Build history of the part. All positions in model axes, mm. A direction names the side the tool comes from. Coordinates: 2 decimals unless noted, no trailing zeros. Order: outer loops, then holes, each group sorted by start corner. A loop starts at its lowest first (then second) coordinate and runs counter-clockwise, first axis right, second up. Notation, with made-up numbers: M -8,-25.5 L -4,-25.5 A21 cw -4,-4.5 Z; hole C 81,9.25 d11. An arc over 180 degrees is marked long. Use a Markdown table: item, result. Add a question column.
from build123d import *

# Parameters (mm, degrees)
F0_R     = 57.15
F1_DEPTH = 14.224
F3_DEPTH = 30.226
F4_R     = 7.112
F5_DEPTH = 0.127


with BuildPart() as f1:
    # F0 (on Top) → F1 (new body)
    with BuildSketch(Plane.XY):
        Circle(F0_R)
        with BuildLine():
            ThreePointArc((0, -29.464), (5.0289434278, -31.5470565722), (7.112, -36.576))
            ThreePointArc((7.112, -36.576), (-5.0289434278, -41.6049434278), (0, -29.464))
        make_face(mode=Mode.SUBTRACT)
        with BuildLine():
            ThreePointArc((-24.5637451688, 18.288), (-24.8060806923, 16.4472789512), (-25.5165724971, 14.732))
            ThreePointArc((-25.5165724971, 14.732), (-38.5454096454, 20.1287210488), (-24.5637451688, 18.288))
        make_face(mode=Mode.SUBTRACT)
        with BuildLine():
            ThreePointArc((15.875, 0), (11.2253201513, -11.2253201513), (0, -15.875))
            ThreePointArc((0, -15.875), (-13.7481532851, -7.9375), (-13.7481532851, 7.9375))
            ThreePointArc((-13.7481532851, 7.9375), (0, 15.875), (13.7481532851, 7.9375))
            ThreePointArc((13.7481532851, 7.9375), (15.3340724923, 4.108752341), (15.875, 0))
        make_face(mode=Mode.SUBTRACT)
        with BuildLine():
            ThreePointArc((38.7877451688, 18.288), (33.5164662176, 11.4183355234), (25.5165724971, 14.732))
            ThreePointArc((25.5165724971, 14.732), (29.8350241201, 25.1576644766), (38.7877451688, 18.288))
        make_face(mode=Mode.SUBTRACT)
    extrude(amount=F1_DEPTH)

    # F2 (on face) → F3 (join)
    with BuildSketch(Plane.XY.offset(14.224)):
        with BuildLine():
            ThreePointArc((-17.1202854359, -34.0368304428), (-32.4337237695, -19.9915872918), (-38.1, 0))
            Line((-38.1, 0), (-50.8, 0))
            ThreePointArc((-50.8, 0), (-43.244965026, -26.6554497224), (-22.8270472479, -45.3824405904))
            Line((-22.8270472479, -45.3824405904), (-17.1202854359, -34.0368304428))
        make_face()
        with BuildLine():
            ThreePointArc((-20.7239090963, 31.9707615137), (0, 38.1), (20.7239090963, 31.9707615137))
            Line((20.7239090963, 31.9707615137), (27.6318787951, 42.6276820183))
            ThreePointArc((27.6318787951, 42.6276820183), (0, 50.8), (-27.6318787951, 42.6276820183))
            Line((-27.6318787951, 42.6276820183), (-20.7239090963, 31.9707615137))
        make_face()
        with BuildLine():
            ThreePointArc((38.1, 0), (32.6002459501, -19.7188732942), (17.6887682944, -33.7448881496))
            Line((17.6887682944, -33.7448881496), (23.5850243925, -44.9931841994))
            ThreePointArc((23.5850243925, -44.9931841994), (43.4669946002, -26.2918310589), (50.8, 0))
            Line((50.8, 0), (38.1, 0))
        make_face()
    extrude(amount=F3_DEPTH)

    # F4 (on face) → F5 (cut)
    with BuildSketch(Plane.XY.offset(14.224)):
        with BuildLine():
            ThreePointArc((-20.7239090963, 31.9707615137), (-47.4729372454, 10.6979144605), (-14.1497451688, 18.288))
            ThreePointArc((-14.1497451688, 18.288), (-15.8785530923, 25.8780855395), (-20.7239090963, 31.9707615137))
        make_face()
        with Locations((-31.6757451688, 18.288)):
            Circle(F4_R, mode=Mode.SUBTRACT)
        with BuildLine():
            ThreePointArc((49.2017451688, 18.288), (39.2658307083, 34.0851920765), (20.7239090963, 31.9707615137))
            ThreePointArc((20.7239090963, 31.9707615137), (24.0856596293, 2.4908079235), (49.2017451688, 18.288))
        make_face()
        with Locations((31.6757451688, 18.288)):
            Circle(F4_R, mode=Mode.SUBTRACT)
        with BuildLine():
            ThreePointArc((-17.4173370009, -34.6273985025), (-0.9758144603, -54.0748131637), (17.526, -36.576))
            ThreePointArc((17.526, -36.576), (1.3253891442, -19.1001875835), (-17.325537101, -33.9328125))
            ThreePointArc((-17.325537101, -33.9328125), (-17.2229897955, -33.9849764235), (-17.1202854359, -34.0368304428))
            Line((-17.1202854359, -34.0368304428), (-17.4173370009, -34.6273985025))
        make_face()
        with Locations((0, -36.576)):
            Circle(F4_R, mode=Mode.SUBTRACT)
    extrude(amount=-F5_DEPTH, mode=Mode.SUBTRACT)


solid = f1.part
(1) Slice it at B-B on y = -14. Give the cut face in (x, z), and give its area (3 significant figures).
(2) Slice it at C-C on x = 11. Give the cut face in (y, z), and give its area (3 significant figures).
(3) Drill centre lines: line 1 along Z through (x, y) = (41, 25); line 2 along X through (y, z) = (-3, 3.5); line 3 along X through (y, z) = (-17, 22). Where is each one in solid material? Low to high. Write a range as from..to.
(4) Slice it at D-D on y = 21.5. Give the cut face in (x, z).
(5) Which spindle directions (+Z, -Z, +X, -X, +Y, -Y) get a long thin tool onto all of the face, cutting with end or side? Do faces 1 (the cylindrical face through (-43.45, -26.32, 29.13)), 2 (the flat face through (45, 0, 29)), 3 (the flat face through (-38, -22, 44.45)), 4 (the cylindrical face through (0.4, 50.8, 29.1)), 5 (the flat face through (8, -36, 14.097)). Say none if no direction does.
(6) Slice it at A-A on z = 22. Give the cut face in (x, y).
(7) Mould opens along X. For faces 6 (the flat face through (20.6, -39.3, 29.1)), 7 (the cylindrical face through (43.266, -26.622, 29.125)), 8 (the flat face through (-24.226, 37.374, 29.125)), 9 (the flat face through (12, -12, 14.224)) say: released by +X, released by -X, zero draft, split by the parting line, or undercut.
(8) Drop flat-ended pins along their axis: P1, Ø1.5, axis at x = -24.5, z = 37, coming from the +Y side; P2, Ø10, axis at x = -44.5, z = 33.5, coming from the +Y side; P3, Ø6, axis at y = -15, z = 30.5, coming from the -X side. Give the stop position or say it passes through.
Solutions:
| question | item | result |
|---|---|---|
| 1 | outline | M -55.41,0 L -7.48,0 L -7.48,14.22 L -35.43,14.22 L -35.43,44.45 L -48.83,44.45 L -48.83,14.22 L -55.41,14.22 Z; M 7.48,0 L 55.41,0 L 55.41,14.22 L 48.83,14.22 L 48.83,44.45 L 35.43,44.45 L 35.43,14.22 L 7.48,14.22 Z |
| 1 | area | 2,170 mm² |
| 2 | outline | M -56.08,0 L -11.45,0 L -11.45,14.22 L -22.93,14.22 L -22.93,14.1 L -50.22,14.1 L -50.22,14.22 L -56.08,14.22 Z; M 11.45,0 L 56.08,0 L 56.08,14.22 L 49.59,14.22 L 49.59,44.45 L 36.48,44.45 L 36.48,14.22 L 11.45,14.22 Z |
| 2 | area | 1,660 mm² |
| 3 | line 1 | 0..14.1 |
| 3 | line 2 | -57.07..-15.59, 15.59..57.07 |
| 3 | line 3 | -47.87..-34.1, 34.1..47.87 |
| 4 | outline | M -52.95,0 L -38.02,0 L -38.02,14.1 L -48.9,14.1 L -48.9,14.22 L -52.95,14.22 Z; M -25.33,0 L 25.33,0 L 25.33,14.1 L 14.45,14.1 L 14.45,14.22 L -14.45,14.22 L -14.45,14.1 L -25.33,14.1 Z; M 38.02,0 L 52.95,0 L 52.95,14.22 L 48.9,14.22 L 48.9,14.1 L 38.02,14.1 Z |
| 5 | face 1 | +Z, -X, -Y |
| 5 | face 2 | +Z, +X, -X, +Y |
| 5 | face 3 | +Z, +X, -X, +Y, -Y |
| 5 | face 4 | +Z, +Y |
| 5 | face 5 | +Z |
| 6 | outline | M -50.8,0 A50.8 ccw -22.83,-45.38 L -17.12,-34.04 A38.1 cw -38.1,0 Z; M -27.63,42.63 L -20.72,31.97 A38.1 cw 20.72,31.97 L 27.63,42.63 A50.8 ccw Z; M 17.69,-33.74 L 23.59,-44.99 A50.8 ccw 50.8,0 L 38.1,0 A38.1 cw Z |
| 7 | face 6 | undercut |
| 7 | face 7 | released by +X |
| 7 | face 8 | released by -X |
| 7 | face 9 | undercut |
| 8 | P1 | y = 44.91 |
| 8 | P2 | y = 0 |
| 8 | P3 | x = -49.36 |
